from build123d import *

# Parameters (mm, degrees)
SKETCH1_R           = 15.5
SKETCH1_R_2         = 3
BOSS_EXTRUDE1_DEPTH = 3
CUT_EXTRUDE3_START  = -3
CUT_EXTRUDE3_DEPTH  = 3
CIRPATTERN2_COUNT   = 18


with BuildPart() as part:
    # Sketch1 → Boss-Extrude1 (new body)
    with BuildSketch(Plane(origin=(0, 0, 0), x_dir=(1, 0, 0), z_dir=(0, 1, 0))):
        with Locations(Location((0, 0, 0), (0, 0, 270))):
            Circle(SKETCH1_R)
        with Locations(Location((0, 0, 0), (0, 0, 270))):
            Circle(SKETCH1_R_2, mode=Mode.SUBTRACT)
    extrude(amount=BOSS_EXTRUDE1_DEPTH)

    # Sketch3 → Cut-Extrude3 (cut)
    with BuildSketch(Plane(origin=(0, 3, 0), x_dir=(1, 0, 0), z_dir=(0, 1, 0)).offset(CUT_EXTRUDE3_START)):
        with BuildLine():
            ThreePointArc((-1, 12.5), (0, 11.5), (1, 12.5))
            add(Edge.make_bspline(
                [(2.316977637, 15.325847925), (1.117647531, 14.032764815), (1, 12.5)],
                knots=[0, 0, 0, 0.821337086, 0.821337086, 0.821337086], degree=2))
            ThreePointArc((2.316977637, 15.325847925), (0, 15.5), (-2.316977637, 15.325847925))
            add(Edge.make_bspline(
                [(-2.316977637, 15.325847925), (-1.117647531, 14.032764815), (-1, 12.5)],
                knots=[0, 0, 0, 0.821337086, 0.821337086, 0.821337086], degree=2))
        make_face()
    cut_extrude3 = extrude(amount=CUT_EXTRUDE3_DEPTH, mode=Mode.SUBTRACT)

    # CirPattern2: Cut-Extrude3 ×18 about axis
    cirpattern2_axis = Axis((0, 3, 0), (0, 1, 0))
    for i in range(1, CIRPATTERN2_COUNT):
        add(cut_extrude3.rotate(cirpattern2_axis, i * 360 / CIRPATTERN2_COUNT), mode=Mode.SUBTRACT)


solid = part.part
Geometry: final body of the model. Coordinates: model frame, mm. Round coordinates to 2 decimals unless told otherwise and drop trailing zeros. Loops run counter-clockwise (first coordinate to the right, second up) from the corner with the lowest first, then second, coordinate; pieces in that order, holes last. Notation, with made-up numbers: M 43,45.25 L 82,45.25 A10 ccw 82,64.25 Z; hole C 46.5,5.25 d5. An arc over 180 degrees is marked long. Put each result on its own line as item: value. Start each with the question number.
(1) Section query B-B (z = 0). Return loops of the section in (x, y).
(2) Contact query for flat-ended pins moving along their axis: pin 1 Ø1.5 at (x, y) = (-6.5, 1) entering from -Z; pin 2 Ø1.5 at (x, y) = (-7.5, 1) entering from -Z. Output: stop coordinate, or through.
(3) Draft query along X for faces 1 (the face through (0.2, 3, 3.2)), 2 (the face through (7.409, 1.479, 8.796)). Return one class per face: +X half, -X half, draft (parallel to the pull), parting line (faces both ways), or undercut.
(4) Material intervals for line 1 along X through (y, z) = (1.75, 0); line 2 along X through (y, z) = (0.3, -11); line 3 along Z through (x, y) = (11, 1.2), sorted ascending. Write a range as [from, to].
(5) Section query A-A (x = 0). Return loops of the section in (y, z), then the cut area to 3 significant figures.
(6) Section query C-C (z = -6.25). Return loops of the section in (x, y), then the cut area to 3 significant figures.
Findings below:
1. outline: M -15.5,0 L -3,0 L -3,3 L -15.5,3 Z; M 3,0 L 15.5,0 L 15.5,3 L 3,3 Z
2. pin 1: stops at z = -13.52
2. pin 2: stops at z = -13.61
3. face 1: draft
3. face 2: undercut
4. line 1: x = [-15.5, -3], [3, 15.5]
4. line 2: x = [-7.71, -4.94], [-3.61, 3.61], [4.94, 7.71]
4. line 3: z = [-10.14, -7.69], [-5.27, 5.27], [7.69, 10.14]
5. outline: M 0,-11.5 L 3,-11.5 L 3,-3 L 0,-3 Z; M 0,3 L 3,3 L 3,11.5 L 0,11.5 Z
5. area: 51.0 mm2
6. outline: M -9.83,0 L 9.83,0 L 9.83,3 L -9.83,3 Z
6. area: 59.0 mm2
